```python
from build123d import *

# Parameters (mm, degrees)
BOSS_EXTRUDE3_DEPTH = 75
SKETCH2_OUTSIDE_W   = 370.368
SKETCH2_OUTSIDE_H   = 220.368
SKETCH2_OUTSIDE_R   = 12.5
CUT_EXTRUDE1_DEPTH  = 150
BOSS_EXTRUDE4_REACH = 227
SKETCH3_R           = 75
SKETCH4_R           = 37.5
CUT_EXTRUDE2_DEPTH  = 150
SKETCH4_4_R         = 50
SKETCH4_4_R_2       = 37.5
CUT_EXTRUDE3_DEPTH  = 20


with BuildPart() as part:
    # Sketch1 → Boss-Extrude3 (new, symmetric)
    with BuildSketch(Plane.XY):
        with BuildLine():
            Line((-150, 25), (-150, 0))
            Line((-150, 0), (-97.488460856, 0))
            ThreePointArc((-97.488460856, 0), (-91.224995055, 12.990386393), (-83.240615087, 25))
            Line((-83.240615087, 25), (-150, 25))
        make_face()
        with BuildLine():
            ThreePointArc((-83.240615087, 25), (-91.224995055, 12.990386393), (-97.488460856, 0))
            Line((-97.488460856, 0), (-69.84983894, 0))
            ThreePointArc((-69.84983894, 0), (-60.236169654, 13.646024213), (-48, 25))
            Line((-48, 25), (-83.240615087, 25))
        make_face()
        with BuildLine():
            ThreePointArc((48, 25), (60.236169654, 13.646024213), (69.84983894, 0))
            Line((69.84983894, 0), (97.488460856, 0))
            ThreePointArc((97.488460856, 0), (91.224995055, 12.990386393), (83.240615087, 25))
            Line((83.240615087, 25), (48, 25))
        make_face()
        with BuildLine():
            ThreePointArc((83.240615087, 25), (0, 66), (-83.240615087, 25))
            Line((-83.240615087, 25), (-48, 25))
            ThreePointArc((-48, 25), (0, 41), (48, 25))
            Line((48, 25), (83.240615087, 25))
        make_face()
        with BuildLine():
            Line((150, 25), (83.240615087, 25))
            ThreePointArc((83.240615087, 25), (91.224995055, 12.990386393), (97.488460856, 0))
            Line((97.488460856, 0), (150, 0))
            Line((150, 0), (150, 25))
        make_face()
    extrude(amount=BOSS_EXTRUDE3_DEPTH, both=True)

    # Sketch2 outside → Cut-Extrude1 (cut)
    # profile 1 of 3: a face of its own
    with BuildSketch(Plane(origin=(0, 0, 0), x_dir=(1, 0, 0), z_dir=(0, 1, 0))):
        Rectangle(SKETCH2_OUTSIDE_W, SKETCH2_OUTSIDE_H)
        with BuildLine():
            Line((-135, -22.912878475), (-30, -68.738635424))
            ThreePointArc((-30, -68.738635424), (0, -75), (30, -68.738635424))
            Line((30, -68.738635424), (135, -22.912878475))
            ThreePointArc((135, -22.912878475), (150, 0), (135, 22.912878475))
            Line((135, 22.912878475), (30, 68.738635424))
            ThreePointArc((30, 68.738635424), (0, 75), (-30, 68.738635424))
            Line((-30, 68.738635424), (-135, 22.912878475))
            ThreePointArc((-135, 22.912878475), (-150, 0), (-135, -22.912878475))
        make_face(mode=Mode.SUBTRACT)
    # profile 2 of 3: a face of its own
    with BuildSketch(Plane(origin=(0, 0, 0), x_dir=(1, 0, 0), z_dir=(0, 1, 0))):
        with Locations(Location((125, 0, 0), (0, 0, 180))):
            Circle(SKETCH2_OUTSIDE_R)
    # profile 3 of 3: a face of its own
    with BuildSketch(Plane(origin=(0, 0, 0), x_dir=(1, 0, 0), z_dir=(0, 1, 0))):
        with Locations(Location((-125, 0, 0), (0, 0, 90))):
            Circle(SKETCH2_OUTSIDE_R)
    extrude(amount=CUT_EXTRUDE1_DEPTH, mode=Mode.SUBTRACT)

    # Sketch3 → Boss-Extrude4 (add, up to next)
    with BuildSketch(Plane(origin=(0, 150, 0), x_dir=(1, 0, 0), z_dir=(0, 1, 0)), mode=Mode.PRIVATE) as boss_extrude4_sk1:
        with Locations(Location((0, 0, 0), (0, 0, 66.421821522))):
            Circle(SKETCH3_R)
    boss_extrude4_tool1 = extrude(boss_extrude4_sk1.sketch, amount=-BOSS_EXTRUDE4_REACH, mode=Mode.PRIVATE) - part.part
    add(boss_extrude4_tool1.solids().sort_by_distance((0, 150, 0))[0])

    # Sketch4 → Cut-Extrude2 (cut)
    with BuildSketch(Plane(origin=(0, 150, 0), x_dir=(1, 0, 0), z_dir=(0, 1, 0))):
        with Locations(Location((0, 0, 0), (0, 0, 270))):
            Circle(SKETCH4_R)
    extrude(amount=-CUT_EXTRUDE2_DEPTH, mode=Mode.SUBTRACT)

    # Sketch4_4 → Cut-Extrude3 (cut)
    with BuildSketch(Plane(origin=(0, 150, 0), x_dir=(1, 0, 0), z_dir=(0, 1, 0))):
        with Locations(Location((0, 0, 0), (0, 0, 270))):
            Circle(SKETCH4_4_R)
        with Locations(Location((0, 0, 0), (0, 0, 270))):
            Circle(SKETCH4_4_R_2, mode=Mode.SUBTRACT)
    extrude(amount=-CUT_EXTRUDE3_DEPTH, mode=Mode.SUBTRACT)


solid = part.part
```
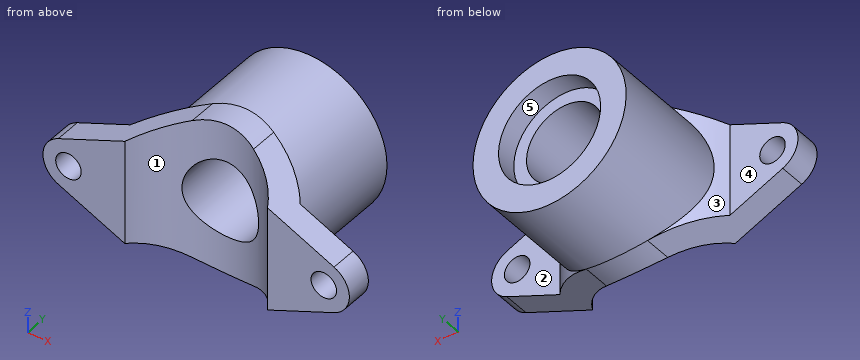
Could you check a few things on this model? Use its own coordinates, in mm. Face numbers are marked on the shaded views. A direction names the side the tool comes from. Round coordinates to 2 decimals unless told otherwise and drop trailing zeros. Loops run counter-clockwise (first coordinate to the right, second up) from the corner with the lowest first, then second, coordinate; pieces in that order, holes last. Notation, with made-up numbers: (21, 72.25) - (50, 72.25) arc R11 ccw to (50, 82.25) - close; hole circle Ø8 at (55.25, 83.5). An arc over 180 degrees is marked (long way). Answer in a Markdown table with one row per item. Add a question column.
(1) For the marked faces 1, 2, 3, 4 and 5, which set-ups out of +Z, -Z, +X, -X, +Y, -Y let a thin tool reach every point of the face, with its end or its side?
(2) I need wall thicknesses on line 1 along X through (y, z) = (99, 0); line 2 along X through (y, z) = (20, 0); line 3 along X through (y, z) = (16, 0). Which ranges of each line are inside material? Lowest first, please.
(3) If we section it at B-B (x = -125): Please give me the cut outline in (y, z), plus the area to 3 significant figures.
(4) I'm going to push flat-ended pins straight in: pin 1 (3 mm diameter, centred on y = 111, z = -44, fed in from +X); pin 2 (1.5 mm diameter, centred on x = 46.5, z = 20, fed in from -Y); pin 3 (4 mm diameter, centred on y = 99, z = 51.5, fed in from -X). Where does each tip first touch, or does it pass through?
(5) If we section it at D-D (z = -29.5): Please give me the cut outline in (x, y), plus the area to 3 significant figures.
(6) If we section it at A-A (z = 0): Please give me the cut outline in (x, y).
(7) If we section it at C-C (y = 11): Please give me the cut outline in (x, z), plus the area to 3 significant figures.
Model answer:
| question | item | result |
|---|---|---|
| 1 | face 1 | +Z, -Z, -Y |
| 1 | face 2 | +Z, -Z, +X, +Y |
| 1 | face 3 | -X, +Y |
| 1 | face 4 | +Z, -Z, -X, +Y |
| 1 | face 5 | +Y |
| 2 | line 1 | x = -75 to -37.5, 37.5 to 75 |
| 2 | line 2 | x = -150 to -137.5, -112.5 to -54.03, 54.03 to 112.5, 137.5 to 150 |
| 2 | line 3 | x = -150 to -137.5, -112.5 to -58.09, 58.09 to 112.5, 137.5 to 150 |
| 3 | outline | (0, -27.28) - (25, -27.28) - (25, -12.5) - (0, -12.5) - close; (0, 12.5) - (25, 12.5) - (25, 27.28) - (0, 27.28) - close |
| 3 | area | 739 mm² |
| 4 | pin 1 | stops at x = 61.8 |
| 4 | pin 2 | stops at y = 25.56 |
| 4 | pin 3 | stops at x = -56.34 |
| 5 | outline | (-119.91, 0) - (-69.85, 0) arc R80 cw to (-23.15, 37.58) - (-23.15, 130) - (-40.37, 130) - (-40.37, 150) - (-68.95, 150) - (-68.95, 40.18) arc R105 ccw to (-83.24, 25) - (-119.91, 25) - close; (23.15, 37.58) arc R80 cw to (69.85, 0) - (119.91, 0) - (119.91, 25) - (83.24, 25) arc R105 ccw to (68.95, 40.18) - (68.95, 150) - (40.37, 150) - (40.37, 130) - (23.15, 130) - close |
| 5 | area | 13,600 mm² |
| 6 | outline | (-150, 0) - (-137.5, 0) - (-137.5, 25) - (-150, 25) - close; (-112.5, 0) - (-69.85, 0) arc R80 cw to (-37.5, 31.67) - (-37.5, 130) - (-50, 130) - (-50, 150) - (-75, 150) - (-75, 34.48) arc R105 ccw to (-83.24, 25) - (-112.5, 25) - close; (37.5, 31.67) arc R80 cw to (69.85, 0) - (112.5, 0) - (112.5, 25) - (83.24, 25) arc R105 ccw to (75, 34.48) - (75, 150) - (50, 150) - (50, 130) - (37.5, 130) - close; (137.5, 0) - (150, 0) - (150, 25) - (137.5, 25) - close |
| 7 | outline | (-135, -22.91) - (-62.45, -54.58) - (-62.45, 54.58) - (-135, 22.91) arc R25 ccw to start; (62.45, -54.58) - (135, -22.91) arc R25 ccw to (135, 22.91) - (62.45, 54.58) - close; hole circle Ø25 at (-125, 0); hole circle Ø25 at (125, 0) |
| 7 | area | 11,300 mm² |
